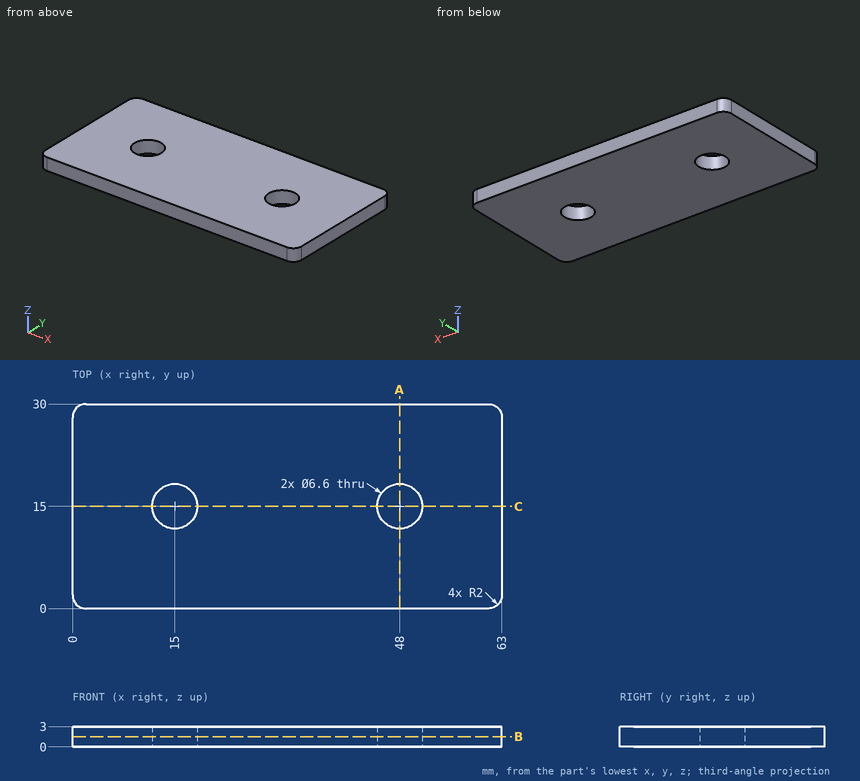
Print and shaded views of the part. All mm, measured from the part's lowest x, y and z. Coordinates: 2 decimals unless noted, no trailing zeros. Loops run counter-clockwise (first coordinate to the right, second up) from the corner with the lowest first, then second, coordinate; pieces in that order, holes last. Notation, with made-up numbers: (-12.75, -29.75) - (13.25, -29.75) arc R20 cw to (13.25, 3.25) - close; hole circle Ø5 at (70.25, -15). An arc over 180 degrees is marked (long way). Write item = value, one per line. Start each with the question number.
Item 1: Wall check: probe 1 along X at (y, z) = (15, 1.9); probe 2 along X at (y, z) = (15.75, 1.5); probe 3 along Y at (x, z) = (48, 0.6). Give the ranges that are in metal, low to high. Write a range as [from, to].
Item 2: Saw through at C-C, the plane y = 15. List the corners of the cut face in (x, z), then the cut area to 3 significant figures.
Item 3: Saw through at B-B, the plane z = 1.5. List the corners of the cut face in (x, y).
Item 4: Saw through at A-A, the plane x = 48. List the corners of the cut face in (y, z), then the cut area to 3 significant figures.
Item 5: Drop flat-ended pins along their axis: pin 1 Ø1.5 at (y, z) = (11, 1) entering from -X; pin 2 Ø4 at (x, y) = (48, 15) entering from -Z. Give the stop position or say it passes through.
Answers:
q1.probe_1 = [0, 11.7], [18.3, 44.7], [51.3, 63]
q1.probe_2 = [0, 11.79], [18.21, 44.79], [51.21, 63]
q1.probe_3 = [0, 11.7], [18.3, 30]
q2.outline = (0, 0) - (11.7, 0) - (11.7, 3) - (0, 3) - close; (18.3, 0) - (44.7, 0) - (44.7, 3) - (18.3, 3) - close; (51.3, 0) - (63, 0) - (63, 3) - (51.3, 3) - close
q2.area = 149 mm2
q3.outline = (0, 2) arc R2 ccw to (2, 0) - (61, 0) arc R2 ccw to (63, 2) - (63, 28) arc R2 ccw to (61, 30) - (2, 30) arc R2 ccw to (0, 28) - close; hole circle Ø6.6 at (15, 15); hole circle Ø6.6 at (48, 15)
q4.outline = (0, 0) - (11.7, 0) - (11.7, 3) - (0, 3) - close; (18.3, 0) - (30, 0) - (30, 3) - (18.3, 3) - close
q4.area = 70.2 mm2
q5.pin_1 = 0
q5.pin_2 = through
